Read the model definition and answer for the solid it produces. Units are mm, in the model's axes. A direction names the side the tool comes from. Give positions to 0.01 mm unless a question says otherwise; leave off trailing zeros. Loops run counter-clockwise (first coordinate to the right, second up) from the corner with the lowest first, then second, coordinate; pieces in that order, holes last. Notation, with made-up numbers: (9.5, 71.5) -> (66.5, 71.5) arc R18 ccw to (66.5, 94.5) -> close; hole circle Ø10 at (79, 6.5). An arc over 180 degrees is marked (long way). Return JSON: item names as keys, results as strings. Group by question number.
from build123d import *

# Parameters (mm, degrees)
SKETCH1_W           = 103.124
SKETCH1_H           = 83.185
BOSS_EXTRUDE1_DEPTH = 25.4
CUT_EXTRUDE1_DEPTH  = 22.225
SKETCH3_W           = 11
SKETCH3_H           = 83.185
CUT_EXTRUDE2_DEPTH  = 12.3
CUT_EXTRUDE3_REACH  = 136.905
SKETCH4_W           = 21.8
SKETCH4_H           = 11.1
SKETCH4_W_2         = 25.1
SKETCH4_H_2         = 12.3
SKETCH6_W           = 46.085
SKETCH6_H           = 9.2
CUT_EXTRUDE5_DEPTH  = 5.08
SKETCH7_W           = 3
SKETCH7_H           = 12
CUT_EXTRUDE6_DEPTH  = 3.175
SKETCH8_W           = 11.1125
SKETCH8_H           = 5.55625
CUT_EXTRUDE7_DEPTH  = 5.08
FILLET1_R           = 4
CUT_EXTRUDE8_REACH  = 136.905
SKETCH9_W           = 21
SKETCH9_H           = 12.3
FILLET2_R           = 0.5


with BuildPart() as part:
    # Sketch1 → Boss-Extrude1 (new body)
    with BuildSketch(Plane(origin=(0, 0, 0), x_dir=(1, 0, 0), z_dir=(0, 1, 0))):
        with Locations((51.562, 41.5925)):
            Rectangle(SKETCH1_W, SKETCH1_H)
    extrude(amount=BOSS_EXTRUDE1_DEPTH)

    # Sketch2 → Cut-Extrude1 (cut)
    with BuildSketch(Plane(origin=(0, 25.4, 0), x_dir=(1, 0, 0), z_dir=(0, 1, 0))):
        Polygon((5, 78.185), (82, 78.185), (82, 69.0118), (87, 69.0118), (87, 5), (12.7, 5), (12.7, 11.7), (5, 11.7), align=None)
    extrude(amount=-CUT_EXTRUDE1_DEPTH, mode=Mode.SUBTRACT)

    # Sketch3 → Cut-Extrude2 (cut)
    with BuildSketch(Plane(origin=(0, 25.4, 0), x_dir=(1, 0, 0), z_dir=(0, 1, 0))):
        with Locations((97.624, 41.5925)):
            Rectangle(SKETCH3_W, SKETCH3_H)
    extrude(amount=-CUT_EXTRUDE2_DEPTH, mode=Mode.SUBTRACT)

    # Sketch4 → Cut-Extrude3 (cut, up to next)
    with BuildSketch(Plane(origin=(0, 0, -83.185), x_dir=(-1, 0, 0), z_dir=(0, 0, -1)), mode=Mode.PRIVATE) as cut_extrude3_sk1:
        with Locations((-71.1, 19.85)):
            Rectangle(SKETCH4_W, SKETCH4_H)
    cut_extrude3_tool1 = extrude(cut_extrude3_sk1.sketch, amount=-CUT_EXTRUDE3_REACH, mode=Mode.PRIVATE) & part.part
    # Sketch4 → Cut-Extrude3 (cut, up to next)
    with BuildSketch(Plane(origin=(0, 0, -83.185), x_dir=(-1, 0, 0), z_dir=(0, 0, -1)), mode=Mode.PRIVATE) as cut_extrude3_sk2:
        with Locations((-20.65, 19.25)):
            Rectangle(SKETCH4_W_2, SKETCH4_H_2)
    cut_extrude3_tool2 = extrude(cut_extrude3_sk2.sketch, amount=-CUT_EXTRUDE3_REACH, mode=Mode.PRIVATE) & part.part
    add(cut_extrude3_tool1.solids().sort_by_distance((71.1, 19.85, -83.185))[0], mode=Mode.SUBTRACT)
    add(cut_extrude3_tool2.solids().sort_by_distance((20.65, 19.25, -83.185))[0], mode=Mode.SUBTRACT)

    # Sketch6 → Cut-Extrude5 (cut)
    with BuildSketch(Plane.ZY):
        with Locations((-34.7425, 20.8)):
            Rectangle(SKETCH6_W, SKETCH6_H)
    extrude(amount=-CUT_EXTRUDE5_DEPTH, mode=Mode.SUBTRACT)

    # Sketch7 → Cut-Extrude6 (cut)
    with BuildSketch(Plane(origin=(0, 25.4, 0), x_dir=(1, 0, 0), z_dir=(0, 1, 0))):
        with Locations((3.5, 63.785)):
            Rectangle(SKETCH7_W, SKETCH7_H)
    extrude(amount=-CUT_EXTRUDE6_DEPTH, mode=Mode.SUBTRACT)

    # Sketch8 → Cut-Extrude7 (cut)
    with BuildSketch(Plane.XZ):
        with Locations((64.23025, -66.119375)):
            Rectangle(SKETCH8_W, SKETCH8_H)
    extrude(amount=-CUT_EXTRUDE7_DEPTH, mode=Mode.SUBTRACT)

    # Fillet1
    fillet1_edges = [part.edges().sort_by_distance(p)[0] for p in [
        (103.124, 6.55, -83.185),
        (103.124, 6.55, 0),
        (0, 12.7, -83.185),
        (0, 12.7, 0),
    ]]
    fillet(fillet1_edges, radius=FILLET1_R)

    # Sketch9 → Cut-Extrude8 (cut, up to next)
    with BuildSketch(Plane.XY, mode=Mode.PRIVATE) as cut_extrude8_sk1:
        with Locations((70.624, 19.25)):
            Rectangle(SKETCH9_W, SKETCH9_H)
    cut_extrude8_tool1 = extrude(cut_extrude8_sk1.sketch, amount=-CUT_EXTRUDE8_REACH, mode=Mode.PRIVATE) & part.part
    add(cut_extrude8_tool1.solids().sort_by_distance((70.624, 19.25, 0))[0], mode=Mode.SUBTRACT)

    # Fillet2
    fillet2_edges = [part.edges().sort_by_distance(p)[0] for p in [
        (5, 19.2125, -57.785),
        (5, 23.8125, -69.785),
        (2, 23.8125, -57.785),
        (2, 23.8125, -69.785),
        (58.674, 1.5875, -68.8975),
        (58.674, 1.5875, -63.34125),
        (69.7865, 1.5875, -63.34125),
        (69.7865, 1.5875, -68.8975),
        (81.124, 19.25, 0),
        (60.124, 19.25, 0),
        (81.124, 19.25, -5),
        (60.124, 19.25, -5),
        (5, 14.2875, -78.185),
        (5, 9.6875, -11.7),
        (12.7, 14.2875, -11.7),
        (12.7, 14.2875, -5),
        (87, 14.2875, -5),
        (87, 14.2875, -69.0118),
        (82, 14.2875, -69.0118),
        (82, 8.7375, -78.185),
        (92.124, 19.25, 0),
        (92.124, 19.25, -83.185),
        (60.2, 19.85, -78.185),
        (82, 19.85, -83.185),
        (60.2, 19.85, -83.185),
        (33.2, 19.25, -78.185),
        (8.1, 19.25, -78.185),
        (33.2, 19.25, -83.185),
        (8.1, 19.25, -83.185),
        (0, 20.8, -11.7),
        (0, 20.8, -57.785),
    ]]
    fillet(fillet2_edges, radius=FILLET2_R)


solid = part.part
1. Section C-C on z = -44 is taken. Determine the outline of the cut face in (x, y) (3 decimals).
2. Which of the six approach directions +Z, -Z, +X, -X, +Y, -Y give full straight-line access (tool end or side, diameter ignored) to faces 1 (the flat face through (33.2, 19, -81)), 2 (the flat face through (70, 13.1, -2)), 3 (the flat face through (69.786, 2, -66)), 4 (the flat face through (50, 14, -5)), 5 (the flat face through (92.124, 19, -41))?
3. Section D-D on x = 24.5 is taken. Determine the outline of the cut face in (y, z) (3 decimals), then the cut area to 3 significant figures.
4. Section A-A on x = 67.5 is taken. Determine the outline of the cut face in (y, z) (1 decimal), then the cut area to 3 significant figures.
5. Straight lines are drawn through the part: line 1 (X direction, y = 3.25, z = -57); line 2 (X direction, y = 13.25, z = -28.5); line 3 (Z direction, x = 46, y = 10.5) (3 decimals). For each, find the intervals that lie inside material, in ascending order. Write a range as from..to.
6. Section B-B on y = 10.5 is taken. Determine the outline of the cut face in (x, z) (3 decimals).
7. Determine the mould class of faces 6 (the flat face through (12.7, 14, -8)), 7 (the flat face through (51, 0, -42)), 8 (the cylindrical face through (101.921, 6.642, -82.044)), 9 (the flat face through (51, 13, 0)) for opening direction Z: pulls with the +Z half, pulls with the -Z half, needs draft (parallel to the pull), parting line crosses it, or undercut.
8. Flat-ended cylindrical pins translate along their axes: pin 1 Ø8 at (y, z) = (22, -23) entering from +X; pin 2 Ø8 at (x, z) = (56, -29.5) entering from +Y (3 decimals); pin 3 Ø2 at (y, z) = (20.5, -81.5) entering from -X. Find the tip coordinate at first contact, or state that the pin passes through.
Completed:
{
 "1": {"outline": "(0, 0) -> (103.124, 0) -> (103.124, 13.1) -> (92.124, 13.1) -> (92.124, 25.4) -> (87, 25.4) -> (87, 3.175) -> (5, 3.175) -> (5, 16.2) -> (0, 16.2) -> close"},
 "2": {"face 1": "-Z, +Y", "face 2": "+Z, +Y", "face 3": "+Y, -Y", "face 4": "+Y", "face 5": "+Z, -Z, +X, +Y"},
 "3": {"outline": "(0, -83.185) -> (13.1, -83.185) -> (13.1, -78.185) -> (3.175, -78.185) -> (3.175, -5) -> (25.4, -5) -> (25.4, 0) -> (0, 0) -> close", "area": "425 mm²"},
 "4": {"outline": "(0, -83.2) -> (14.3, -83.2) -> (14.3, -78.2) -> (3.2, -78.2) -> (3.2, -68.9) -> (0, -68.9) -> close; (0, -63.3) -> (3.2, -63.3) -> (3.2, -5) -> (13.1, -5) -> (13.1, 0) -> (0, 0) -> close", "area": "352 mm²"},
 "5": {"line 1": "x = 0..5, 87..103.12", "line 2": "x = 0..5, 87..92.12", "line 3": "z = -83.185..-78.185, -5..0"},
 "6": {"outline": "(0, -79.185) arc R4 ccw to (4, -83.185) -> (99.124, -83.185) arc R4 ccw to (103.124, -79.185) -> (103.124, -4) arc R4 ccw to (99.124, 0) -> (4, 0) arc R4 ccw to (0, -4) -> close; hole (5, -77.685) arc R0.5 ccw to (5.5, -78.185) -> (81.5, -78.185) arc R0.5 ccw to (82, -77.685) -> (82, -69.512) arc R0.5 cw to (82.5, -69.012) -> (86.5, -69.012) arc R0.5 ccw to (87, -68.512) -> (87, -5.5) arc R0.5 ccw to (86.5, -5) -> (13.2, -5) arc R0.5 ccw to (12.7, -5.5) -> (12.7, -11.2) arc R0.5 cw to (12.2, -11.7) -> (5.5, -11.7) arc R0.5 ccw to (5, -12.2) -> close"},
 "7": {"face 6": "undercut", "face 7": "needs draft", "face 8": "pulls with the -Z half", "face 9": "pulls with the +Z half"},
 "8": {"pin 1": "stops at x = 92.12", "pin 2": "stops at y = 3.175", "pin 3": "stops at x = 0.22"}
}
